For this review, take the finished solid that the model builds, in its own axes (mm). A direction names the side the tool comes from. Coordinates: 2 decimals unless noted, no trailing zeros. Loops run counter-clockwise (first coordinate to the right, second up) from the corner with the lowest first, then second, coordinate; pieces in that order, holes last. Notation, with made-up numbers: M 11.25,-32 L 34.25,-32 A35 ccw 34.25,2 Z; hole C 59,-2 d6. An arc over 180 degrees is marked long. Use one line per item in the form item = value.
```python
from build123d import *

# Parameters (mm, degrees)
ESBO_O1_R                = 11
ESBO_O1_R_2              = 6
RESSALTO_EXTRUS_O1_DEPTH = 50.8
CORTE_EXTRUS_O1_START    = -5.85
ESBO_O2_R                = 11
ESBO_O2_R_2              = 10.5
CORTE_EXTRUS_O1_DEPTH    = 1.3
CORTE_EXTRUS_O2_START    = -4.55
ESBO_O3_R                = 11
ESBO_O3_R_2              = 10.5
CORTE_EXTRUS_O2_DEPTH    = 1.3
FILETE1_R                = 0.5


with BuildPart() as part:
    # Esboço1 → Ressalto-extrusão1 (new body)
    with BuildSketch(Plane(origin=(0, 0, 0), x_dir=(1, 0, 0), z_dir=(0, 1, 0))):
        with Locations(Location((0, 0, 0), (0, 0, 270))):
            Circle(ESBO_O1_R)
        with Locations(Location((0, 0, 0), (0, 0, 270))):
            Circle(ESBO_O1_R_2, mode=Mode.SUBTRACT)
    extrude(amount=RESSALTO_EXTRUS_O1_DEPTH)

    # Esboço2 → Corte-extrusão1 (cut)
    with BuildSketch(Plane(origin=(0, 50.8, 0), x_dir=(1, 0, 0), z_dir=(0, 1, 0)).offset(CORTE_EXTRUS_O1_START)):
        with Locations(Location((0, 0, 0), (0, 0, 270))):
            Circle(ESBO_O2_R)
        with Locations(Location((0, 0, 0), (0, 0, 270))):
            Circle(ESBO_O2_R_2, mode=Mode.SUBTRACT)
    extrude(amount=CORTE_EXTRUS_O1_DEPTH, mode=Mode.SUBTRACT)

    # Esboço3 → Corte-extrusão2 (cut)
    with BuildSketch(Plane.XZ.offset(CORTE_EXTRUS_O2_START)):
        with Locations(Location((0, 0, 0), (0, 0, 270))):
            Circle(ESBO_O3_R)
        with Locations(Location((0, 0, 0), (0, 0, 90))):
            Circle(ESBO_O3_R_2, mode=Mode.SUBTRACT)
    extrude(amount=-CORTE_EXTRUS_O2_DEPTH, mode=Mode.SUBTRACT)

    # Filete1
    filete1_edges = [part.edges().sort_by_distance(p)[0] for p in [
        (0, 0, -11),
        (0, 50.8, -11),
    ]]
    fillet(filete1_edges, radius=FILETE1_R)


solid = part.part
```
1. For pin 1 Ø5 at (x, y) = (-4.5, 44) entering from +Z; pin 2 Ø2 at (y, z) = (44, 8.5) entering from +X; pin 3 Ø8 at (y, z) = (10, -6) entering from -X, all flat-tipped, find the tip position at first contact; note any pin that passes through.
Computed values:
pin_1 = 10.82
pin_2 = 8.05
pin_3 = -10.82
2. Tool access review of faces 4 (the face through (-5, 0, 5)), 5 (the face through (-4, 5.85, -10)): name each direction out of +Z, -Z, +X, -X, +Y, -Y from which nothing blocks a thin tool from reaching the whole face with its end or side.
Computed values:
face_4 = +Z, -Z, +X, -X, -Y
face_5 = none
3. Consider section B-B on y = 29. Write out the cut boundary in (x, z), plus the area to 3 significant figures.
Computed values:
outline = C 0,0 d22; hole C 0,0 d12
area = 267 mm2
4. Draft analysis for pull direction Y (two halves, no side actions). For faces 1 (the face through (-5, 50.8, 5)), 2 (the face through (1.802, 25.044, 5.723)), 3 (the face through (-4, 46.25, 10)), state which applies: +Y half, -Y half, draft (parallel to the pull), parting line (faces both ways), or undercut.
Computed values:
face_1 = +Y half
face_2 = draft
face_3 = undercut
5. Consider section A-A on x = 0. Write out the cut boundary in (y, z), plus the area to 3 significant figures.
Computed values:
outline = M 0,-10.5 A0.5 ccw 0.5,-11 L 4.55,-11 L 4.55,-10.5 L 5.85,-10.5 L 5.85,-11 L 44.95,-11 L 44.95,-10.5 L 46.25,-10.5 L 46.25,-11 L 50.3,-11 A0.5 ccw 50.8,-10.5 L 50.8,-6 L 0,-6 Z; M 0,6 L 50.8,6 L 50.8,10.5 A0.5 ccw 50.3,11 L 46.25,11 L 46.25,10.5 L 44.95,10.5 L 44.95,11 L 5.85,11 L 5.85,10.5 L 4.55,10.5 L 4.55,11 L 0.5,11 A0.5 ccw 0,10.5 Z
area = 505 mm2
6. Wall thickness on line 1 along X through (y, z) = (33, 0); line 2 along X through (y, z) = (46, 0); line 3 along Z through (x, y) = (5.5, 25.5): over which ranges is each line inside the solid? List them lowest first. Write a range as from..to.
Computed values:
line_1 = -11..-6, 6..11
line_2 = -10.5..-6, 6..10.5
line_3 = -9.53..-2.4, 2.4..9.53
